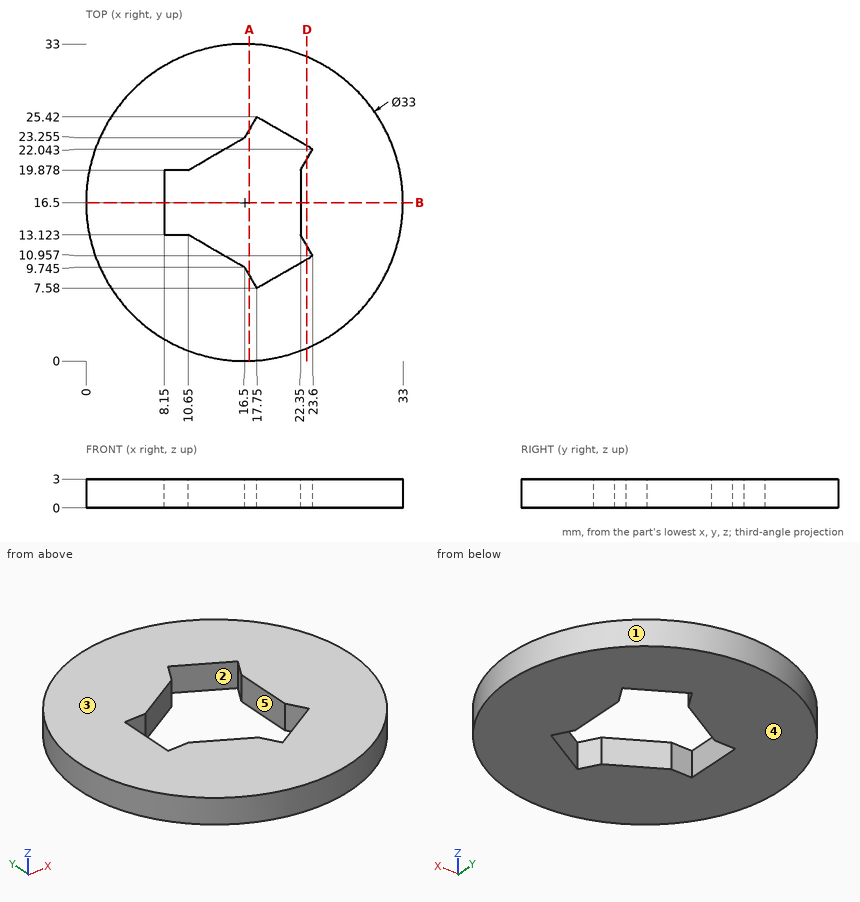
The drawing under review shows one solid part. Ordinate dimensions are in mm from its lowest x, y, z. A direction names the side the tool comes from. Give positions to 0.01 mm unless a question says otherwise; leave off trailing zeros. Write each loop counter-clockwise with the first axis right and the second up, starting at its lowest first coordinate (ties: lowest second). Pieces come first, ordered by that corner, then holes.
1. Add section B-B, the plane y = 16.5. Write out the cut boundary in (x, z), plus the area to 3 significant figures.
2. Wall thickness on L1, parallel to Y at x = 23, z = 2.7 (1 decimal); L2, parallel to X at y = 21, z = 0.55 (1 decimal); L3, parallel to Y at x = 20, z = 2.7 (1 decimal): over which ranges is each line inside the solid? List them lowest first.
3. Add section D-D, the plane x = 23. Write out the cut boundary in (y, z) (1 decimal).
4. Tool access review of the marked faces 4 and 5: name each direction out of +Z, -Z, +X, -X, +Y, -Y from which nothing blocks a thin tool from reaching the whole face with its end or side.
5. Draft analysis for pull direction Y (two halves, no side actions). For the marked faces 1, 2 and 3, state which applies: +Y half, -Y half, draft (parallel to the pull), parting line (faces both ways), or undercut.
6. For P1, Ø0.9, axis at y = 17.5, z = 1.5, coming from the -X side; P2, Ø5, axis at x = 18, y = 12.5, coming from the -Z side; P3, Ø0.8, axis at x = 9, z = 1, coming from the -Y side (1 decimal); P4, Ø1, axis at y = 8.5, z = 2.5, coming from the +X side, all flat-tipped, find the tip position at first contact; note any pin that passes through.
7. Add section A-A, the plane x = 17. Write out the cut boundary in (y, z).
Worked answers:
1. outline: (0, 0) - (8.15, 0) - (8.15, 3) - (0, 3) - close; (22.35, 0) - (33, 0) - (33, 3) - (22.35, 3) - close
1. area: 56.4 mm2
2. L1: y = 1.3 to 10.6, 12 to 21, 22.4 to 31.7
2. L2: x = 0.6 to 12.6, 23 to 32.4
2. L3: y = 0.4 to 8.9, 24.1 to 32.6
3. outline: (1.3, 0) - (10.6, 0) - (10.6, 3) - (1.3, 3) - close; (12, 0) - (21, 0) - (21, 3) - (12, 3) - close; (22.4, 0) - (31.7, 0) - (31.7, 3) - (22.4, 3) - close
4. face 4: -Z, +X, -X, +Y, -Y
4. face 5: +Z, -Z
5. face 1: parting line
5. face 2: undercut
5. face 3: draft
6. P1: stops at x = 0.01
6. P2: passes through
6. P3: stops at y = 1.6
6. P4: stops at x = 31.2
7. outline: (0.01, 0) - (8.88, 0) - (8.88, 3) - (0.01, 3) - close; (24.12, 0) - (32.99, 0) - (32.99, 3) - (24.12, 3) - close
